from build123d import *

# Parameters (mm, degrees)
F0_R     = 10.668
F0_R_2   = 6.6675
F1_DEPTH = 254
F2_SIZE2 = 5.08
F2_SIZE  = 2.54
F3_R     = 0.508
F4_R     = 0.508


with BuildPart() as f1:
    # F0 (on Front) → F1 (new body)
    with BuildSketch(Plane.XZ):
        Circle(F0_R)
        Circle(F0_R_2, mode=Mode.SUBTRACT)
    extrude(amount=F1_DEPTH)

    # F2
    f2_edges = [f1.edges().sort_by_distance(p)[0] for p in [
        (-6.6675, 0, 0),
    ]]
    f2_side = f1.faces().sort_by_distance((-10.366263, 0, 0))[0]
    chamfer(f2_edges, length=F2_SIZE, length2=F2_SIZE2, reference=f2_side)

    # F3
    f3_edges = [f1.edges().sort_by_distance(p)[0] for p in [
        (-10.668, 0, 0),
        (-9.2075, 0, 0),
    ]]
    fillet(f3_edges, radius=F3_R)

    # F4
    f4_edges = [f1.edges().sort_by_distance(p)[0] for p in [
        (-10.668, -254, 0),
        (-6.6675, -254, 0),
    ]]
    fillet(f4_edges, radius=F4_R)


solid = f1.part
Read the model definition and answer for the solid it produces. Units are mm, in the model's axes. Round coordinates to 2 decimals unless told otherwise and drop trailing zeros. Loops run counter-clockwise (first coordinate to the right, second up) from the corner with the lowest first, then second, coordinate; pieces in that order, holes last.
Q1. Each of these flat-tipped pins is pushed along its axis until it touches: pin 1 (4 mm diameter, centred on x = -0.5, z = 4.5, fed in from -Y); pin 2 (3 mm diameter, centred on x = -6, y = -216, fed in from +Z); pin 3 (2 mm diameter, centred on x = -4, y = -75.5, fed in from +Z); pin 4 (1.5 mm diameter, centred on x = 7.5, z = 4, fed in from +Y). Where does it stop, or does it pass through?
Q2. Section A-A on x = 0 is taken. Write down the section's boundary in (y, z), and give its area (3 significant figures).
Q3. Consider probe 1 along Z at (x, y) = (0, -134.5); probe 2 along X at (y, z) = (-190, -0.25); probe 3 along X at (y, z) = (-108, 2). Determine where each line is inside the solid, lowest interval first.
Q4. Section B-B on z = 0 is taken. Write down the section's boundary in (x, y), and give its area (3 significant figures).
Q5. Section C-C on y = -46 is taken. Write down the section's boundary in (x, z) (1 decimal), and give its area (3 significant figures).
Q6. Determine the mould class of faces 1 (the face through (-0.87, -127.55, 6.61)), 2 (the face through (-0.883, -4.847, 6.726)), 3 (the face through (4, -254, -7)), 4 (the face through (4.923, -125.229, -9.464)) for opening direction X: released by +X, released by -X, zero draft, split by the parting line, or undercut.
Output:
1. pin 1: passes through
1. pin 2: stops at z = 9.67
1. pin 3: stops at z = 10.24
1. pin 4: stops at y = -0.08
2. outline: (-254, -10.16) arc R0.51 ccw to (-253.49, -10.67) - (-0.51, -10.67) arc R0.51 ccw to (0, -10.16) - (0, -9.52) arc R0.51 ccw to (-0.28, -9.07) - (-5.08, -6.67) - (-253.49, -6.67) arc R0.51 ccw to (-254, -7.18) - close; (-254, 7.18) arc R0.51 ccw to (-253.49, 6.67) - (-5.08, 6.67) - (-0.28, 9.07) arc R0.51 ccw to (0, 9.52) - (0, 10.16) arc R0.51 ccw to (-0.51, 10.67) - (-253.49, 10.67) arc R0.51 ccw to (-254, 10.16) - close
2. area: 2,020 mm2
3. probe 1: z = -10.67 to -6.67, 6.67 to 10.67
3. probe 2: x = -10.67 to -6.66, 6.66 to 10.67
3. probe 3: x = -10.48 to -6.36, 6.36 to 10.48
4. outline: (-10.67, -253.49) arc R0.51 ccw to (-10.16, -254) - (-7.18, -254) arc R0.51 ccw to (-6.67, -253.49) - (-6.67, -5.08) - (-9.07, -0.28) arc R0.51 ccw to (-9.52, 0) - (-10.16, 0) arc R0.51 ccw to (-10.67, -0.51) - close; (6.67, -253.49) arc R0.51 ccw to (7.18, -254) - (10.16, -254) arc R0.51 ccw to (10.67, -253.49) - (10.67, -0.51) arc R0.51 ccw to (10.16, 0) - (9.52, 0) arc R0.51 ccw to (9.07, -0.28) - (6.67, -5.08) - close
4. area: 2,020 mm2
5. outline: circle Ø21.3 at (0, 0); hole circle Ø13.3 at (0, 0)
5. area: 218 mm2
6. face 1: undercut
6. face 2: undercut
6. face 3: zero draft
6. face 4: split by the parting line
